Geometry: see drawing. Coordinates: mm, zero at the bounding-box minimum. Coordinates: 2 decimals unless noted, no trailing zeros. Loops run counter-clockwise (first coordinate to the right, second up) from the corner with the lowest first, then second, coordinate; pieces in that order, holes last. Notation, with made-up numbers: (-25.5, -33) - (-7.5, -33) arc R23 cw to (-7.5, -23) - close; hole circle Ø7 at (3, 60.25). An arc over 180 degrees is marked (long way). Use one line per item in the form item = value.
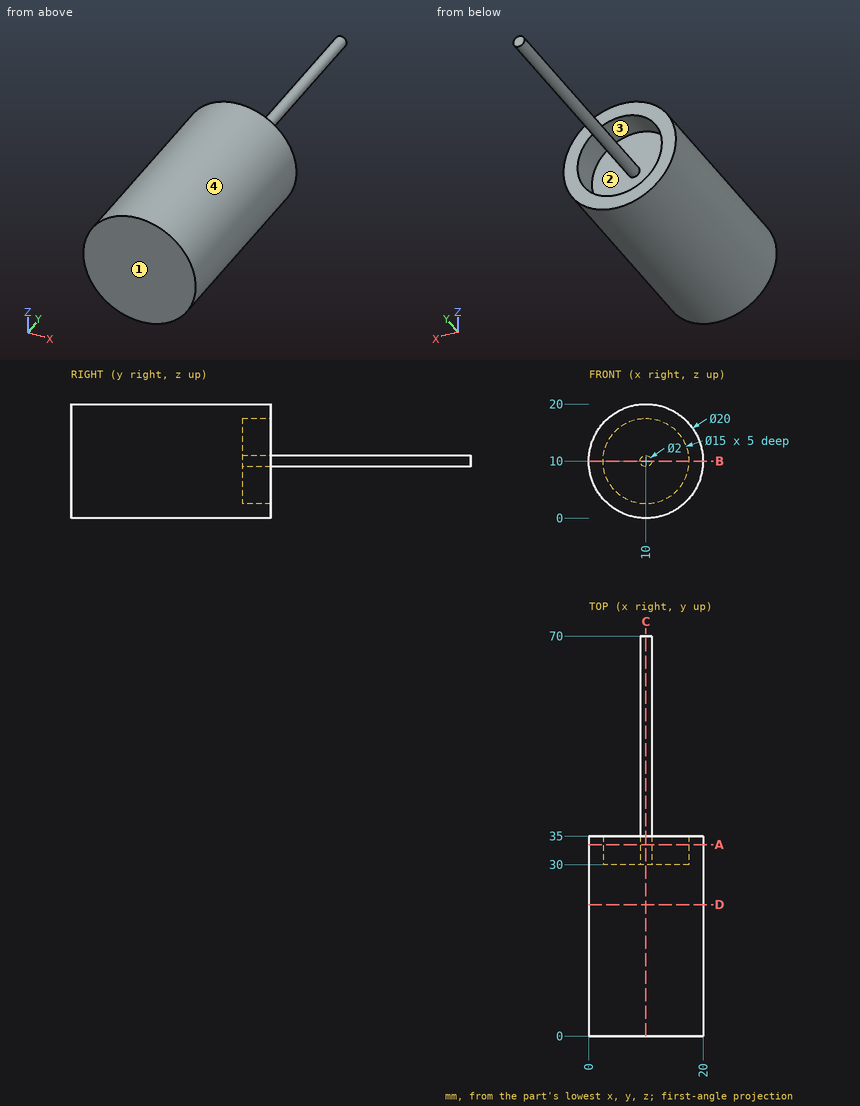
Q1. Cut plane C-C, the plane x = 10. Return loops of the section in (y, z), then the cut area to 3 significant figures.
Check values:
outline = (0, 0) - (35, 0) - (35, 2.5) - (30, 2.5) - (30, 9) - (70, 9) - (70, 11) - (30, 11) - (30, 17.5) - (35, 17.5) - (35, 20) - (0, 20) - close
area = 705 mm²
Q2. Cut plane D-D, the plane y = 23. Return loops of the section in (x, z), then the cut area to 3 significant figures.
Check values:
outline = circle Ø20 at (10, 10)
area = 314 mm²
Q3. Cut plane A-A, the plane y = 33.5. Return loops of the section in (x, z).
Check values:
outline = circle Ø20 at (10, 10); circle Ø2 at (10, 10); hole circle Ø15 at (10, 10)
Q4. Ray query, line 1 along X through (y, z) = (33.5, 10); line 2 along Y through (x, z) = (18.75, 11.75); line 3 along Z through (x, y) = (10.5, 10). Return the intervals inside material, ascending. Write a range as [from, to].
Check values:
line_1 = [0, 2.5], [9, 11], [17.5, 20]
line_2 = [0, 35]
line_3 = [0.01, 19.99]
Q5. Pull-direction query (X, two-part tool) for the marked faces 1, 2, 3 and 4; classes: pulls with the +X half, pulls with the -X half, needs draft (parallel to the pull), parting line crosses it, or undercut.
Check values:
face_1 = needs draft
face_2 = undercut
face_3 = undercut
face_4 = parting line crosses it
Q6. First-contact query: P1, Ø4, axis at x = 6, y = 57.5, coming from the -Z side; P2, Ø5, axis at x = 7.5, z = 7.5, coming from the +Y side; P3, Ø1, axis at x = 2.5, y = 23, coming from the +Z side; P4, Ø1, axis at x = 16.5, y = 25.5, coming from the +Z side. Flat tips, straight axial feed; report the tip coordinate or a pass-through.
Check values:
P1 = through
P2 = 30
P3 = 17.14
P4 = 18
Q7. Cut plane B-B, the plane z = 10. Return loops of the section in (x, y), then the cut area to 3 significant figures.
Check values:
outline = (0, 0) - (20, 0) - (20, 35) - (17.5, 35) - (17.5, 30) - (11, 30) - (11, 70) - (9, 70) - (9, 30) - (2.5, 30) - (2.5, 35) - (0, 35) - close
area = 705 mm²
